The listing builds one solid part. Answer for the finished solid, in the listing's coordinates (mm). Face numbers are marked on the shaded views. Give positions to 0.01 mm unless a question says otherwise; leave off trailing zeros. Order: outer loops, then holes, each group sorted by start corner. A loop starts at its lowest first (then second) coordinate and runs counter-clockwise, first axis right, second up. Notation, with made-up numbers: (-34, 89) - (1, 89) arc R10 ccw to (1, 95) - close; hole circle Ø3 at (-31.5, 24). An arc over 180 degrees is marked (long way). Use a Markdown table: item, result. Add a question column.
1) Flat-ended cylindrical pins translate along their axes: pin 1 (6 mm diameter, centred on x = 61.5, z = 6, fed in from +Y); pin 2 (10 mm diameter, centred on x = 25, y = -53.5, fed in from -Z); pin 3 (10 mm diameter, centred on y = -11, z = 9.5, fed in from +X). Find the tip coordinate at first contact, or state that the pin passes through.
2) Find section D-D, the plane y = -77. Determine the outline of the cut face in (x, z), plus the area to 3 significant figures.
3) Find section B-B, the plane z = 35. Determine the outline of the cut face in (x, y), plus the area to 3 significant figures.
4) Find section A-A, the plane y = 0. Determine the outline of the cut face in (x, z), plus the area to 3 significant figures.
5) Straight lines are drawn through the part: line 1 (Y direction, x = 0, z = 15) (3 decimals); line 2 (Z direction, x = 40.5, y = -48.5); line 3 (Y direction, x = -10.5, z = 17). For each, find the intervals that lie inside material, in ascending order.
6) Find section C-C, the plane x = -23. Determine the outline of the cut face in (y, z), plus the area to 3 significant figures.
7) The mould has two halves that part along Y. Classify the marked faces 1, 2 and 3: released by +Y, released by -Y, zero draft, split by the parting line, or undercut.
from build123d import *

# Parameters (mm, degrees)
EXTRUDE_1_DEPTH     = 20
SKETCH_2_R          = 10
CUT_EXTRUDE_1_DEPTH = 20
SKETCH_6_R          = 4
EXTRUDE_3_DEPTH     = 30
SKETCH_7_R          = 4
EXTRUDE_4_DEPTH     = 30


with BuildPart() as part:
    # 草图1 → 凸台-拉伸1 (new body)
    with BuildSketch(Plane.XY):
        with BuildLine():
            Line((-1.176470588, 19.965367939), (-85.882352941, 14.974025955))
            ThreePointArc((-85.882352941, 14.974025955), (-100, 0), (-85.882352941, -14.974025955))
            Line((-85.882352941, -14.974025955), (-18.763483586, -18.92904326))
            ThreePointArc((-18.763483586, -18.92904326), (-12.125205702, -20.924621234), (-7.09296905, -25.691764928))
            Line((-7.09296905, -25.691764928), (65.330255198, -136.407322955))
            ThreePointArc((65.330255198, -136.407322955), (85.671434943, -141.015620535), (90.955210971, -120.839354505))
            Line((90.955210971, -120.839354505), (17.42945106, 9.80888555))
            ThreePointArc((17.42945106, 9.80888555), (9.582712413, 17.554817653), (-1.176470588, 19.965367939))
        make_face()
    extrude(amount=EXTRUDE_1_DEPTH)

    # 草图2 → 切除-拉伸1 (cut)
    with BuildSketch(Plane.XY):
        Circle(SKETCH_2_R)
    extrude(amount=CUT_EXTRUDE_1_DEPTH, mode=Mode.SUBTRACT)

    # 草图6 → 凸台-拉伸3 (add)
    with BuildSketch(Plane.XY.offset(20)):
        with Locations((-85, 0)):
            Circle(SKETCH_6_R)
    extrude(amount=EXTRUDE_3_DEPTH)

    # 草图7 → 凸台-拉伸4 (add)
    with BuildSketch(Plane(origin=(0, 0, 0), x_dir=(-1, 0, 0), z_dir=(0, 0, -1))):
        with Locations(Location((-77.883122675, -128.196018668, 0), (0, 0, 180))):
            Circle(SKETCH_7_R)
    extrude(amount=EXTRUDE_4_DEPTH)


solid = part.part
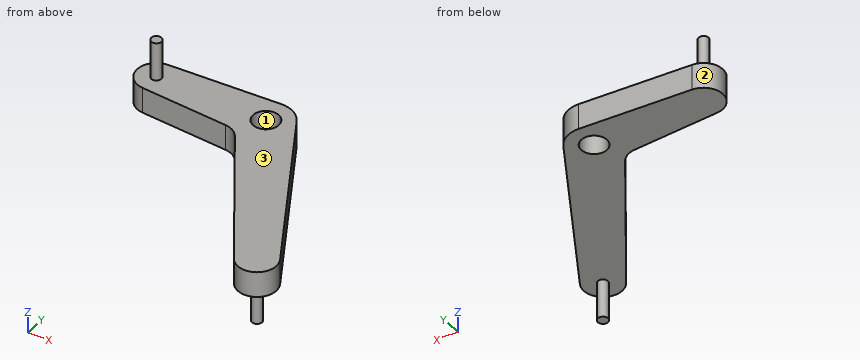
The answers:
| question | item | result |
|---|---|---|
| 1 | pin 1 | y = -63.17 |
| 1 | pin 2 | z = 0 |
| 1 | pin 3 | x = 31.95 |
| 2 | outline | (26.47, 0) - (66.28, 0) - (66.28, 20) - (26.47, 20) - close |
| 2 | area | 796 mm2 |
| 3 | outline | circle Ø8 at (-85, 0) |
| 3 | area | 50.3 mm2 |
| 4 | outline | (-100, 0) - (-10, 0) - (-10, 20) - (-81, 20) - (-81, 50) - (-89, 50) - (-89, 20) - (-100, 20) - close; (10, 0) - (22.95, 0) - (22.95, 20) - (10, 20) - close |
| 4 | area | 2,300 mm2 |
| 5 | line 1 | -36.535 to -10, 10 to 20 |
| 5 | line 2 | 0 to 20 |
| 5 | line 3 | -22.01 to 19.42 |
| 6 | outline | (-18.68, 0) - (18.68, 0) - (18.68, 20) - (-18.68, 20) - close |
| 6 | area | 747 mm2 |
| 7 | face 1 | undercut |
| 7 | face 2 | split by the parting line |
| 7 | face 3 | zero draft |
